Print and shaded views of the part. All mm, measured from the part's lowest x, y and z. Round coordinates to 2 decimals unless told otherwise and drop trailing zeros. Write each loop counter-clockwise with the first axis right and the second up, starting at its lowest first coordinate (ties: lowest second). Pieces come first, ordered by that corner, then holes. Notation, with made-up numbers: M -15,-14 L 4,-14 A29 cw 4,7 Z; hole C 8,-39 d3. An arc over 180 degrees is marked long. Write item = value, one per line. Start each with the question number.
Q1. Band-saw the part on B-B on z = 4. Write the cut outline in (x, y), plus the area to 3 significant figures.
Q2. Band-saw the part on C-C on y = 0.95. Write the cut outline in (x, z) (3 decimals).
Q3. Pull direction Z, two halves, no side cores. Call the marked faces 1, 2 and 3: released by +Z, released by -Z, zero draft, split by the parting line, or undercut.
Q4. Probe L1, parallel to Z at x = 3, y = 0.75 (3 decimals); L2, parallel to Z at x = 4, y = 2.3; L3, parallel to X at y = 0.25, z = 12.5. List the from-to ranges inside material, lowest first.
Q5. Band-saw the part on A-A on x = 3. Write the cut outline in (y, z) (3 decimals), plus the area to 3 significant figures.
Q6. Band-saw the part on D-D on x = 2.3. Write the cut outline in (y, z).
Q7. Drop flat-ended pins along their axis: P1, Ø1, axis at x = 1.5, y = 1.5, coming from the +Z side; P2, Ø1.5, axis at x = 1, y = 2, coming from the -Z side; P3, Ø3.5, axis at x = 3, z = 3, coming from the -Y side. Give the stop position or say it passes through.
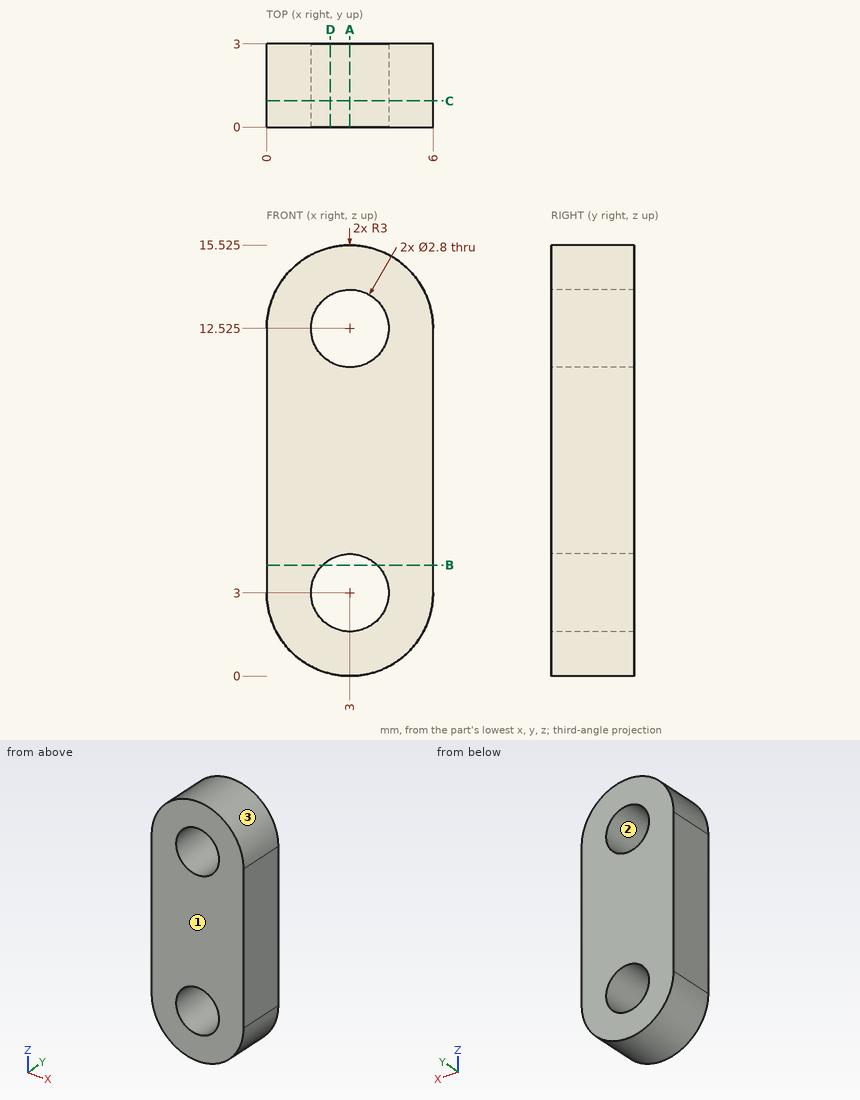
Conclusion:
q1.outline = M 0,0 L 2.02,0 L 2.02,3 L 0,3 Z; M 3.98,0 L 6,0 L 6,3 L 3.98,3 Z
q1.area = 12.1 mm^2
q2.outline = M 0,3 A3 ccw 6,3 L 6,12.525 A3 ccw 0,12.525 Z; hole C 3,3 d2.8; hole C 3,12.525 d2.8
q3.face_1 = zero draft
q3.face_2 = undercut
q3.face_3 = released by +Z
q4.L1 = 0 to 1.6, 4.4 to 11.125, 13.925 to 15.525
q4.L2 = 0.17 to 2.02, 3.98 to 11.55, 13.5 to 15.35
q4.L3 = 0 to 1.6, 4.4 to 6
q5.outline = M 0,0 L 3,0 L 3,1.6 L 0,1.6 Z; M 0,4.4 L 3,4.4 L 3,11.125 L 0,11.125 Z; M 0,13.925 L 3,13.925 L 3,15.525 L 0,15.525 Z
q5.area = 29.8 mm^2
q6.outline = M 0,0.08 L 3,0.08 L 3,1.79 L 0,1.79 Z; M 0,4.21 L 3,4.21 L 3,11.31 L 0,11.31 Z; M 0,13.74 L 3,13.74 L 3,15.44 L 0,15.44 Z
q7.P1 = 15.35
q7.P2 = 0.27
q7.P3 = 0
